Can you work these out from the drawing? Everything is in mm from the part's minimum corner. A direction names the side the tool comes from. Coordinates: 2 decimals unless noted, no trailing zeros. Loops run counter-clockwise (first coordinate to the right, second up) from the corner with the lowest first, then second, coordinate; pieces in that order, holes last. Notation, with made-up numbers: (64.25, 40.25) - (79.25, 40.25) arc R13 ccw to (79.25, 51.25) - close; hole circle Ø6 at (-5, 37.5). An arc over 180 degrees is marked (long way). Use CSV: the item, a comma, the result in double quotes.
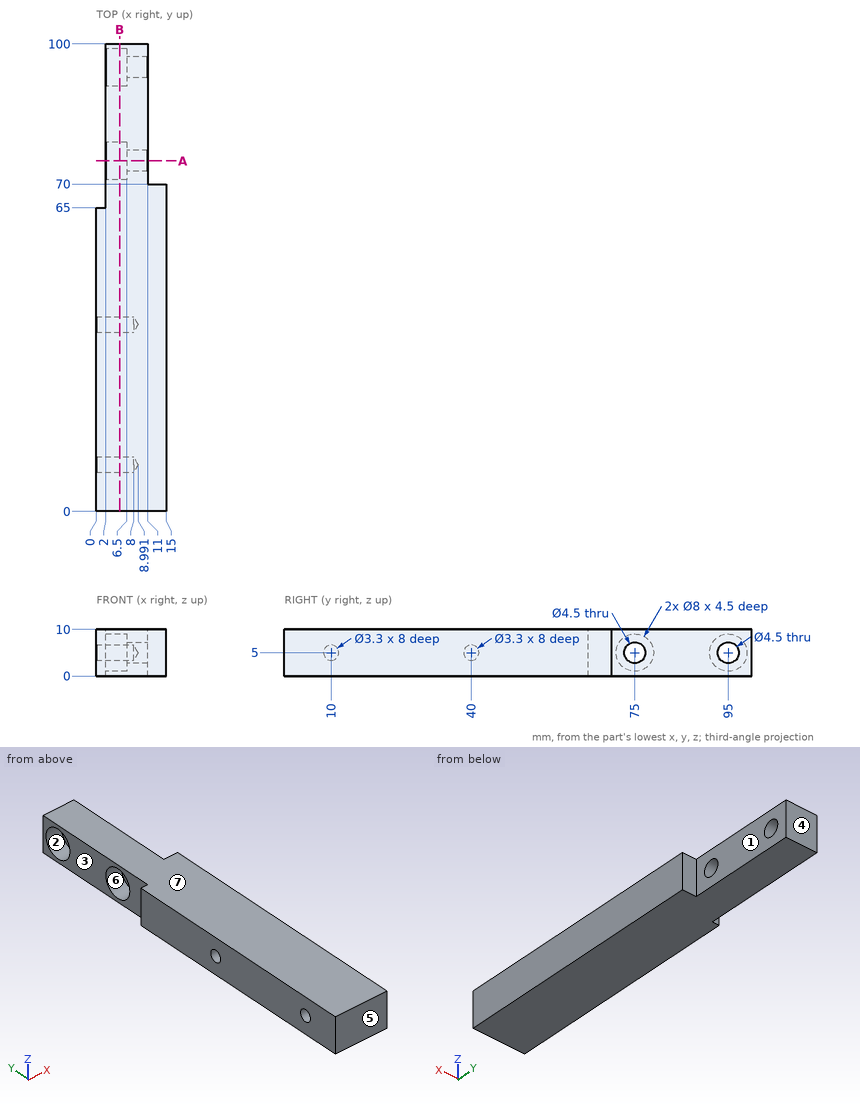
(1) Will these pins go through, and if not, where does the flat tip stop? pin 1 (5 mm diameter, centred on y = 95, z = 5, fed in from -X); pin 2 (5 mm diameter, centred on x = 13, y = 51, fed in from -Z); pin 3 (3 mm diameter, centred on y = 87, z = 6, fed in from +X); pin 4 (2 mm diameter, centred on y = 10, z = 5, fed in from -X).
Computed:
pin 1,"stops at x = 6.5"
pin 2,"stops at z = 0"
pin 3,"stops at x = 11"
pin 4,"stops at x = 8.39"
(2) Suppose I cut it at A-A (y = 75). Write out the boundary of the cut face in (x, z).
Computed:
outline,"(2, 0) - (11, 0) - (11, 2.75) - (6.5, 2.75) - (6.5, 1) - (2, 1) - close; (2, 9) - (6.5, 9) - (6.5, 7.25) - (11, 7.25) - (11, 10) - (2, 10) - close"
(3) Which directions (+Z, -Z, +X, -X, +Y, -Y) give clear straight access to the entire face, cutting with the end or side of a thin tool? Please do the marked faces 1, 2, 3 and 4.
Computed:
face 1,"+Z, -Z, +X, +Y"
face 2,"-X"
face 3,"+Z, -Z, -X, +Y"
face 4,"+Z, -Z, +X, -X, +Y"
(4) Suppose I cut it at B-B (x = 5). Write out the boundary of the cut face in (y, z).
Computed:
outline,"(0, 0) - (100, 0) - (100, 10) - (0, 10) - close; hole circle Ø3.3 at (10, 5); hole circle Ø3.3 at (40, 5); hole circle Ø8 at (75, 5); hole circle Ø8 at (95, 5)"
(5) Thinking about a two-plate mould opening in Z: for the marked faces 5, 6 and 7, which applies, +Z half, -Z half, draft (parallel to the pull), parting line (faces both ways), or undercut?
Computed:
face 5,"draft"
face 6,"undercut"
face 7,"+Z half"
(6) Please list where these lines run through material, in increasing order: line 1 (Y direction, x = 6, z = 5); line 2 (Z direction, x = 9, y = 75); line 3 (Y direction, x = 10.05, z = 5).
Computed:
line 1,"y = 0 to 8.35, 11.65 to 38.35, 41.65 to 71, 79 to 91, 99 to 100"
line 2,"z = 0 to 2.75, 7.25 to 10"
line 3,"y = 0 to 72.75, 77.25 to 92.75, 97.25 to 100"
